For this review, take the finished solid that the model builds, in its own axes (mm). Face numbers are marked on the shaded views. Coordinates: 2 decimals unless noted, no trailing zeros.
1) To check wall thickness, follow line 1 along X through (y, z) = (-44.5, 12.25); line 2 along X through (y, z) = (-31.5, 14.5); line 3 along Z through (x, y) = (-13, -31). State the ranges of each line that lie inside material, in increasing order.
2) Insertion check: P1, Ø2, axis at y = 5.5, z = 1.5, coming from the -X side; P2, Ø2, axis at x = 0.5, z = 1.5, coming from the +Y side; P3, Ø2, axis at y = -10, z = 1.5, coming from the -X side. Each pin has a flat end and moves straight along its axis. Give the tip position at first contact, or say it passes through.
3) Mouldability with a two-part tool opening along Y and no side actions: class the marked faces 1 and 2 as pulls with the +Y half, pulls with the -Y half, needs draft (parallel to the pull), parting line crosses it, or undercut.
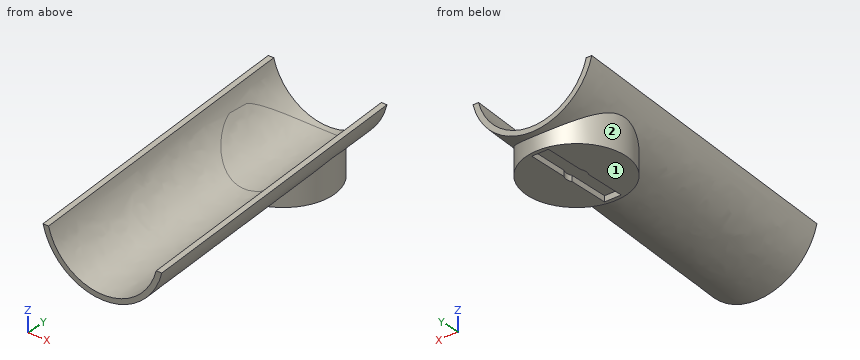
from build123d import *

# Parameters (mm, degrees)
SKETCH1_R           = 17.5
BOSS_EXTRUDE1_DEPTH = 15
CUT_EXTRUDE1_DEPTH  = 2
SKETCH9_R           = 20
CUT_EXTRUDE2_DEPTH  = 100.381983754


with BuildPart() as part:
    # Sketch1 → Boss-Extrude1 (new body)
    with BuildSketch(Plane.XY):
        Circle(SKETCH1_R)
    extrude(amount=BOSS_EXTRUDE1_DEPTH)

    # Sketch2 → Cut-Extrude1 (cut)
    with BuildSketch(Plane(origin=(0, 0, 0), x_dir=(-1, 0, 0), z_dir=(0, 0, -1))):
        with BuildLine():
            Line((3, 1.802775638), (3, 16.1))
            Line((3, 16.1), (-3, 16.1))
            Line((-3, 16.1), (-3, 1.802775638))
            ThreePointArc((-3, 1.802775638), (-3.5, 0), (-3, -1.802775638))
            Line((-3, -1.802775638), (-3, -16.1))
            Line((-3, -16.1), (3, -16.1))
            Line((3, -16.1), (3, -1.802775638))
            ThreePointArc((3, -1.802775638), (3.5, 0), (3, 1.802775638))
        make_face()
    extrude(amount=-CUT_EXTRUDE1_DEPTH, mode=Mode.SUBTRACT)

    # Sweep1: sweep along a path in Sketch8
    with BuildLine(Plane(origin=(0, 0, 0), x_dir=(0, 0, -1), z_dir=(1, 0, 0))) as sweep1_path:
        Line((-5.24788844, 19.5), (3.467685835, -80.119469809))
    # Sketch5 → Sweep1 (sweep)
    with BuildSketch(Plane(origin=(0, 19.5, 0), x_dir=(1, 0, 0), z_dir=(0, 1, 0))):
        with BuildLine():
            Line((-21.364916731, -22), (-19.364916731, -22))
            ThreePointArc((-19.364916731, -22), (0, -7), (19.364916731, -22))
            Line((19.364916731, -22), (21.364916731, -22))
            ThreePointArc((21.364916731, -22), (0, -5.24788844), (-21.364916731, -22))
        make_face()
    sweep(path=sweep1_path.line)

    # Sketch9 → Cut-Extrude2 (cut, along a direction that is not the sketch's normal)
    with BuildSketch(Plane(origin=(0, 19.5, 0), x_dir=(1, 0, 0), z_dir=(0, 1, 0))):
        with Locations((0, -27)):
            Circle(SKETCH9_R)
    extrude(amount=-CUT_EXTRUDE2_DEPTH, dir=(0, 0.9961946980917461, 0.08715574274765157), mode=Mode.SUBTRACT)


solid = part.part
Result:
1. line 1: x = -19.89 to -17.78, 17.78 to 19.89
1. line 2: x = -20.38 to -18.31, 18.31 to 20.38
1. line 3: z = 5.08 to 7.38
2. P1: stops at x = -16.91
2. P2: stops at y = 17.5
2. P3: stops at x = -15.01
3. face 1: needs draft
3. face 2: undercut
